Read the model definition and answer for the solid it produces. Units are mm, in the model's axes. Face numbers are marked on the shaded views. Coordinates: 2 decimals unless noted, no trailing zeros. Write each loop counter-clockwise with the first axis right and the second up, starting at its lowest first coordinate (ties: lowest second). Pieces come first, ordered by that corner, then holes. Notation, with made-up numbers: (-2, 28.25) -> (15, 28.25) arc R16 ccw to (15, 34.25) -> close; hole circle Ø4 at (-29, -1.75). An arc over 180 degrees is marked (long way). Answer as a JSON object with one key per item and string values. Group by question number.
(1) Flat-ended cylindrical pins translate along their axes: P1, Ø10, axis at y = 120.5, z = 3.5, coming from the -X side; P2, Ø2, axis at y = 43.5, z = -24, coming from the +X side; P3, Ø2, axis at y = 35.5, z = -14.5, coming from the +X side. Find the tip coordinate at first contact, or state that the pin passes through.
(2) Straight lines are drawn through the part: L1, parallel to X at y = 73, z = 0; L2, parallel to Z at x = -14, y = 145.5; L3, parallel to X at y = 85, z = 8.5. For each, find the intervals that lie inside material, in ascending order.
(3) For a pull along Z with two mould halves and no side action, classify the marked faces 1 and 2 as +Z half, -Z half, draft (parallel to the pull), parting line (faces both ways), or undercut.
(4) Find section B-B (z = 0). Give the vertices of the cut face in (x, y).
(5) Find section A-A (x = 0). Give the vertices of the cut face in (y, z), then the cut area to 3 significant figures.
(6) Find section C-C (y = 165.5). Give the vertices of the cut face in (x, z).
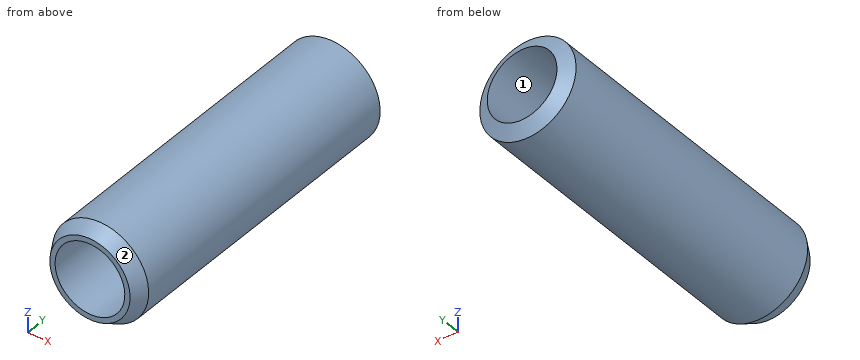
from build123d import *

# Parameters (mm, degrees)
SKETCH1_R           = 30
BOSS_EXTRUDE1_DEPTH = 202.993196
SKETCH2_R           = 21.720790464
CUT_EXTRUDE1_DEPTH  = 208.379453231
CHAMFER1_SIZE       = 4.98909
CHAMFER1_SIZE_2     = 8.641358


with BuildPart() as part:
    # Sketch1 → Boss-Extrude1 (new body)
    with BuildSketch(Plane(origin=(0, 0, 0), x_dir=(1, 0, 0), z_dir=(0, 1, 0))):
        with Locations(Location((0, 0, 0), (0, 0, 270))):
            Circle(SKETCH1_R)
    extrude(amount=BOSS_EXTRUDE1_DEPTH)

    # Sketch2 → Cut-Extrude1 (cut, through all)
    with BuildSketch(Plane(origin=(0, 0, 0), x_dir=(1, 0, 0), z_dir=(0, 1, 0))):
        with Locations(Location((0, 0, 0), (0, 0, 270))):
            Circle(SKETCH2_R)
    extrude(amount=CUT_EXTRUDE1_DEPTH, mode=Mode.SUBTRACT)

    # Chamfer1
    # the kernel refuses this chamfer: 8.641358, 4.98909 mm, written as the material it takes off along each edge
    with BuildSketch(Plane(origin=(0, 202.993196, 0), x_dir=(0, 0, 1), z_dir=(-1, 0, 0))) as chamfer1_piece_1:
        Polygon((30, -CHAMFER1_SIZE), (30 - CHAMFER1_SIZE_2, 0), (30, 0), align=None)
    revolve(axis=Axis((0, 202.993196, 0), (0, 1, 0)), mode=Mode.SUBTRACT)
    with BuildSketch(Plane(origin=(0, 0, 0), x_dir=(0, 0, 1), z_dir=(-1, 0, 0))) as chamfer1_piece_2:
        Polygon((30, CHAMFER1_SIZE_2), (30 - CHAMFER1_SIZE, 0), (30, 0), align=None)
    revolve(axis=Axis((0, 0, 0), (0, 1, 0)), mode=Mode.SUBTRACT)


solid = part.part
Results below:
{
 "1": {"P1": "stops at x = -30", "P2": "stops at x = 19.26", "P3": "stops at x = 26.79"},
 "2": {"L1": "x = -30 to -21.72, 21.72 to 30", "L2": "z = -26.53 to -16.61, 16.61 to 26.53", "L3": "x = -28.77 to -19.99, 19.99 to 28.77"},
 "3": {"face 1": "undercut", "face 2": "parting line"},
 "4": {"outline": "(-30, 8.64) -> (-25.01, 0) -> (-21.72, 0) -> (-21.72, 202.78) -> (-30, 198) -> close; (21.72, 0) -> (25.01, 0) -> (30, 8.64) -> (30, 198) -> (21.72, 202.78) -> close"},
 "5": {"outline": "(0, -25.01) -> (8.64, -30) -> (198, -30) -> (202.78, -21.72) -> (0, -21.72) -> close; (0, 21.72) -> (202.78, 21.72) -> (198, 30) -> (8.64, 30) -> (0, 25.01) -> close", "area": "3,280 mm2"},
 "6": {"outline": "circle Ø60 at (0, 0); hole circle Ø43.44 at (0, 0)"}
}
